```python
from build123d import *

# Parameters (mm, degrees)
F0_W     = 60
F0_H     = 60
F1_DEPTH = 904
F2_D     = 5.5
F4_D     = 5.5


with BuildPart() as f1:
    # F0 (on Right) → F1 (new body)
    with BuildSketch(Plane.YZ):
        with Locations((-30, 30)):
            Rectangle(F0_W, F0_H)
    extrude(amount=F1_DEPTH)

    # F2 (through all)
    with Locations(Plane(origin=(0, 0, 0), x_dir=(0, 1, 0), z_dir=(-1, 0, 0))):
        with Locations((-45, -45), (-45, -15), (-15, -15), (-15, -45)):
            Hole(F2_D / 2)

    # F4 (through all)
    with Locations(Plane.XZ.offset(60)):
        with Locations((150, 45), (150, 15)):
            Hole(F4_D / 2)


solid = f1.part
```
Can you work these out from the model? Positions are in its coordinate system, mm. Give positions to 0.01 mm unless a question says otherwise; leave off trailing zeros. Loops run counter-clockwise (first coordinate to the right, second up) from the corner with the lowest first, then second, coordinate; pieces in that order, holes last. Notation, with made-up numbers: M 43.5,-4.75 L 64.5,-4.75 A19 cw 64.5,20.25 Z; hole C 14.25,22.25 d1. An arc over 180 degrees is marked long. Use CSV: the item, a comma, the result in double quotes. Start each with the question number.
1. For P1, Ø3.5, axis at y = -45, z = 15, coming from the +X side, with a flat end and sliding along its axis, tell me the tip position at first contact or that it passes through.
2. Imagine slicing it at A-A, the plane x = 169. Write out the boundary of the cut face in (y, z).
3. If I drill on L1, parallel to Z at x = 150, y = -3.75; L2, parallel to X at y = -51, z = 15; L3, parallel to Y at x = 643.5, z = 46, over which ranges is the centre line in solid material (lowest first)?
Response values:
1,P1,"through"
2,outline,"M -60,0 L 0,0 L 0,60 L -60,60 Z; hole C -45,15 d5.5; hole C -45,45 d5.5; hole C -15,15 d5.5; hole C -15,45 d5.5"
3,L1,"0 to 12.25, 17.75 to 42.25, 47.75 to 60"
3,L2,"0 to 147.25, 152.75 to 904"
3,L3,"-60 to -47.56, -42.44 to -17.56, -12.44 to 0"
